Autodesk Fusion 360 part; units mm, degrees
sketch "Szkic1" plane through (0, 0, 0) normal (0, 0, 1) x (1, 0, 0)
  line L0 (0, 0) -> (2, 0)
  line L1 (2, 0) -> (3, 1.7321)
  line L2 (3, 1.7321) -> (2, 3.4641)
  line L3 (2, 3.4641) -> (0, 3.4641)
  line L4 (0, 3.4641) -> (-1, 1.7321)
  line L5 (-1, 1.7321) -> (0, 0)
  point P0 (1, 1.7321)
extrude "Wyciągnięcie proste1" add sketch "Szkic1" along normal blind 12
sketch "Szkic2" plane through (0, 0, 12) normal (0, 0, 1) x (-1, 0, 0)
  line L0 (1, -1.7321) -> (0, 0)
  line L1 (0, 0) -> (-2, 0)
  line L2 (-2, 0) -> (-3, -1.7321)
  line L3 (-3, -1.7321) -> (-2, -3.4641)
  line L4 (-2, -3.4641) -> (0, -3.4641)
  line L5 (0, -3.4641) -> (1, -1.7321)
  line L6 (1, -1.7321) -> (0, 0)
  line L7 (0, 0) -> (-2, 0)
  line L8 (-2, 0) -> (-3, -1.7321)
  line L9 (-3, -1.7321) -> (-2, -3.4641)
  line L10 (-2, -3.4641) -> (0, -3.4641)
  line L11 (0, -3.4641) -> (1, -1.7321)
  line L12 (1, -1.7321) -> (-3, -1.7321)
  line L13 (-2, -3.4641) -> (0, 0)
  circle A0 centre (-1, -1.7321) radius 1.1
  dimension "d3" = 2.2
hole "Otwór1" at (1, 1.7321, 12) direction (0, 0, -1) diameter 2.2 end through all
The listing builds one solid part. Answer for the finished solid, in the listing's coordinates (mm). Coordinates: 2 decimals unless noted, no trailing zeros. Loops run counter-clockwise (first coordinate to the right, second up) from the corner with the lowest first, then second, coordinate; pieces in that order, holes last. Notation, with made-up numbers: M 1.5,-7 L 22.5,-7 A33 cw 22.5,23 Z; hole C 33,76 d4. An arc over 180 degrees is marked long. Answer as a JSON object with one key per item and string values. Group by question number.
Item 1: This flat-tipped pin is pushed along its axis until it touches: P1, Ø1, axis at x = 1, y = 2, coming from the -Z side. Where does it stop, or does it pass through?
Item 2: Consider L1, parallel to Y at x = 1, z = 4.25; L2, parallel to Y at x = 0.55, z = 1; L3, parallel to X at y = 1.95, z = 10. Determine where each line is inside the solid, lowest interval first.
Item 3: Section B-B (z = 1.75) is taken. Write down the section's boundary in (x, y).
Item 4: Determine the mould class of faces 1 (the face through (-0.09, 1.88, 5.92)), 2 (the face through (1, 3.464, 6)), 3 (the face through (-0.51, 0.88, 5.92)) for opening direction X: +X half, -X half, draft (parallel to the pull), parting line (faces both ways), or undercut.
Item 5: Section A-A (x = 1) is taken. Write down the section's boundary in (y, z).
Item 6: Section C-C (y = 1.3) is taken. Write down the section's boundary in (x, z), and give its area (3 significant figures).
Solved:
{
 "1": {"P1": "passes through"},
 "2": {"L1": "y = 0 to 0.63, 2.83 to 3.46", "L2": "y = 0 to 0.73, 2.74 to 3.46", "L3": "x = -0.87 to -0.08, 2.08 to 2.87"},
 "3": {"outline": "M -1,1.73 L 0,0 L 2,0 L 3,1.73 L 2,3.46 L 0,3.46 Z; hole C 1,1.73 d2.2"},
 "4": {"face 1": "undercut", "face 2": "draft", "face 3": "-X half"},
 "5": {"outline": "M 0,0 L 0.63,0 L 0.63,12 L 0,12 Z; M 2.83,0 L 3.46,0 L 3.46,12 L 2.83,12 Z"},
 "6": {"outline": "M -0.75,0 L -0.01,0 L -0.01,12 L -0.75,12 Z; M 2.01,0 L 2.75,0 L 2.75,12 L 2.01,12 Z", "area": "17.7 mm2"}
}
